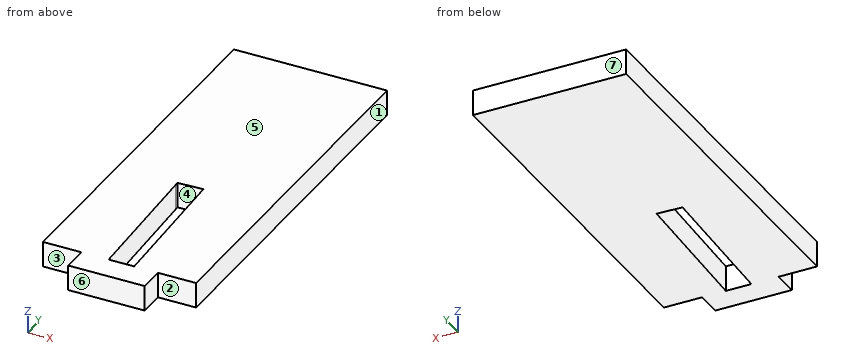
```python
from build123d import *

# Parameters (mm, degrees)
EXTRUDE_1_DEPTH     = 2
SKETCH_3_W          = 12
SKETCH_3_H          = 1.078774048
CUT_EXTRUDE_2_DEPTH = 10
CUT_EXTRUDE_3_DEPTH = 2


with BuildPart() as part:
    # 草图1 → 凸台-拉伸1 (new body)
    with BuildSketch(Plane.XY):
        Polygon((-6, 0), (-6, 15), (-6, 30.078774409), (6, 30.078774409), (6, 15), (6, 0), (3, 0), (3, -2), (-3, -2), (-3, 0), align=None)
    extrude(amount=EXTRUDE_1_DEPTH)

    # 草图3 → 切除-拉伸2 (cut)
    with BuildSketch(Plane.XY.offset(2)):
        with Locations((0, 29.539387385)):
            Rectangle(SKETCH_3_W, SKETCH_3_H)
        Polygon((6, 29.000000361), (10.298878861, 29.000000361), (10.298878861, 34.143483695), (-9.585000786, 34.143483695), (-9.585000786, 29.000000361), (-6, 29.000000361), (-6, 30.078774409), (6, 30.078774409), align=None)
    extrude(amount=-CUT_EXTRUDE_2_DEPTH, mode=Mode.SUBTRACT)

    # 草图4 → 切除-拉伸3 (cut)
    with BuildSketch(Plane.XY.offset(2)):
        Polygon((1.144251734, 0.005791625), (-0.857088089, 0), (-1.291547484, 10.965059679), (-1.305754189, 11.323614176), (0.692677741, 11.402796374), align=None)
    extrude(amount=-CUT_EXTRUDE_3_DEPTH, mode=Mode.SUBTRACT)


solid = part.part
```
For this review, take the finished solid that the model builds, in its own axes (mm). Face numbers are marked on the shaded views. A direction names the side the tool comes from. Coordinates: 2 decimals unless noted, no trailing zeros. Loops run counter-clockwise (first coordinate to the right, second up) from the corner with the lowest first, then second, coordinate; pieces in that order, holes last.
1. For line 1 (Y direction, x = 4.5, z = 1.9); line 2 (X direction, y = 5, z = 0.6); line 3 (Y direction, x = 0.5, z = 0.4), list the stretches that pass through material, from the lowest coordinate up.
2. Mouldability with a two-part tool opening along Y and no side actions: class the marked faces 4, 5, 6 and 7 as +Y half, -Y half, draft (parallel to the pull), parting line (faces both ways), or undercut.
3. Add section A-A, the plane z = 0.3. Give the boundary of the cut face in (x, y), then the cut area to 3 significant figures.
4. Add section D-D, the plane x = 4.5. Give the boundary of the cut face in (y, z).
5. For the marked faces 1, 2 and 3, list the 3-axis set-ups (+Z, -Z, +X, -X, +Y, -Y) from which the entire face can be reached by the end or side of a thin tool; tool diameter is ignored.
6. Insertion check: P1, Ø0.6, axis at x = -4.5, z = 1, coming from the -Y side; P2, Ø0.6, axis at y = -0.5, z = 1, coming from the -X side. Each pin has a flat end and moves straight along its axis. Give the tip position at first contact, or say it passes through.
7. Add section C-C, the plane y = 6. Give the boundary of the cut face in (x, z).
8. Add section B-B, the plane x = -0.5. Give the boundary of the cut face in (y, z).
Result:
1. line 1: y = 0 to 29
1. line 2: x = -6 to -1.06, 0.95 to 6
1. line 3: y = -2 to 0, 11.4 to 29
2. face 4: undercut
2. face 5: draft
2. face 6: -Y half
2. face 7: +Y half
3. outline: (-6, 0) - (-3, 0) - (-3, -2) - (3, -2) - (3, 0) - (6, 0) - (6, 29) - (-6, 29) - close; hole (-1.31, 11.32) - (-0.86, 0) - (1.14, 0.01) - (0.69, 11.4) - close
3. area: 337 mm2
4. outline: (0, 0) - (29, 0) - (29, 2) - (0, 2) - close
5. face 1: +Z, -Z, +X, +Y, -Y
5. face 2: +Z, -Z, +X, -Y
5. face 3: +Z, -Z, -X, -Y
6. P1: stops at y = 0
6. P2: stops at x = -3
7. outline: (-6, 0) - (-1.09, 0) - (-1.09, 2) - (-6, 2) - close; (0.91, 0) - (6, 0) - (6, 2) - (0.91, 2) - close
8. outline: (-2, 0) - (0, 0) - (0, 2) - (-2, 2) - close; (11.36, 0) - (29, 0) - (29, 2) - (11.36, 2) - close
